Geometry check sheet. Reference: drawing and pictorial views, mm from the part's lowest x, y, z. Round coordinates to 2 decimals unless told otherwise and drop trailing zeros. Order: outer loops, then holes, each group sorted by start corner. A loop starts at its lowest first (then second) coordinate and runs counter-clockwise, first axis right, second up. Notation, with made-up numbers: M -21.5,-26.5 L 11.5,-26.5 A20 ccw 11.5,7.5 Z; hole C 48.25,-10 d8. An arc over 180 degrees is marked long. Answer as a JSON object with one key per item and string values. Group by question number.
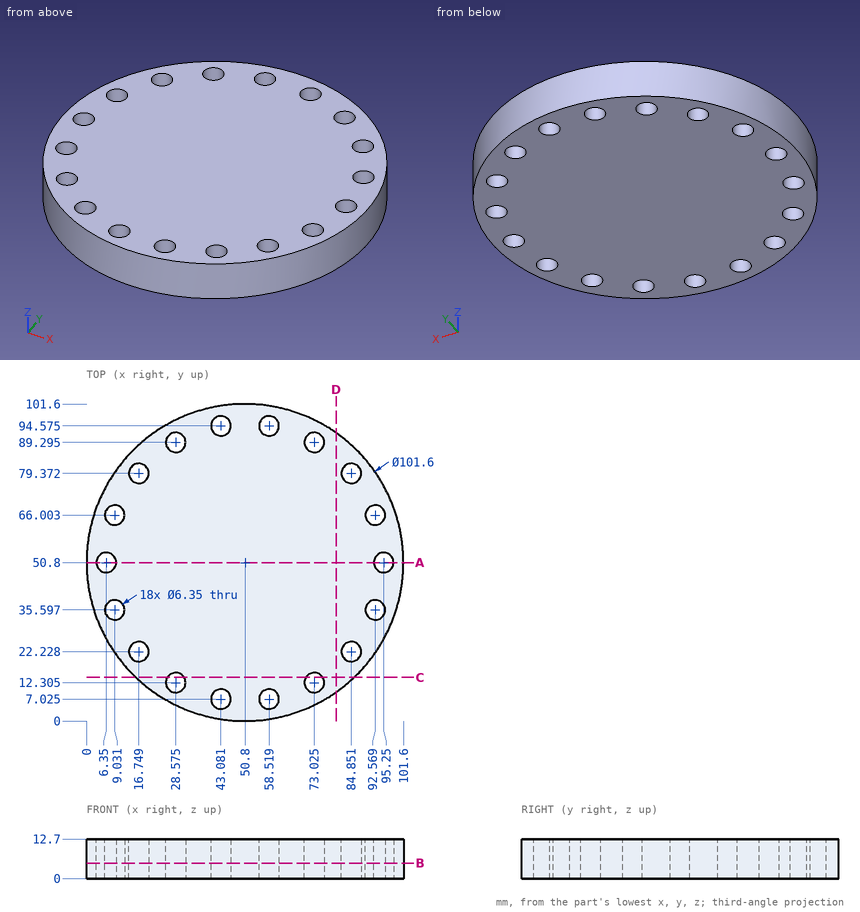
Q1. Thickness scan on line 1 (Y direction, x = 28, z = 6.75) (1 decimal); line 2 (Y direction, x = 44.5, z = 5.5) (1 decimal); line 3 (X direction, y = 80, z = 2). Record the ranges inside material, lowest first. Write a range as from..to.
Q2. Cross-section at D-D, the plane x = 80. Record the cut outline in (y, z).
Q3. Cross-section at A-A, the plane y = 50.8. Record the cut outline in (x, z) (1 decimal).
Q4. Cross-section at C-C, the plane y = 14. Record the cut outline in (x, z), then the cut area to 3 significant figures.
Q5. Gauge pin test, flat ends, axial feed: pin 1 Ø5 at (x, y) = (84.85, 22.23) entering from -Z; pin 2 Ø6 at (x, z) = (90, 7.5) entering from +Y; pin 3 Ø6 at (x, z) = (38, 3.5) entering from -Y; pin 4 Ø1 at (x, z) = (12, 5) entering from +Y. Record the tip position at first contact, or that the pin passes through.
Q6. Cross-section at B-B, the plane z = 5. Give the number of separate pieces and of enclosed holes in the cut face, then the cut area to 3 significant figures.
Conclusion:
{
 "1": {"line 1": "5.4..9.2, 15.4..86.2, 92.4..96.2", "line 2": "0.4..4.2, 9.9..91.7, 97.4..101.2", "line 3": "9.23..13.64, 19.86..81.74, 87.96..92.37"},
 "2": {"outline": "M 9.23,0 L 92.37,0 L 92.37,12.7 L 9.23,12.7 Z"},
 "3": {"outline": "M 0,0 L 3.2,0 L 3.2,12.7 L 0,12.7 Z; M 9.5,0 L 92.1,0 L 92.1,12.7 L 9.5,12.7 Z; M 98.4,0 L 101.6,0 L 101.6,12.7 L 98.4,12.7 Z"},
 "4": {"outline": "M 15.78,0 L 25.89,0 L 25.89,12.7 L 15.78,12.7 Z; M 31.26,0 L 70.34,0 L 70.34,12.7 L 31.26,12.7 Z; M 75.71,0 L 85.82,0 L 85.82,12.7 L 75.71,12.7 Z", "area": "753 mm2"},
 "5": {"pin 1": "through", "pin 2": "y = 86.44", "pin 3": "y = 0.95", "pin 4": "y = 84.17"},
 "6": {"separate pieces": "1", "enclosed holes": "18", "area": "7,540 mm2"}
}
